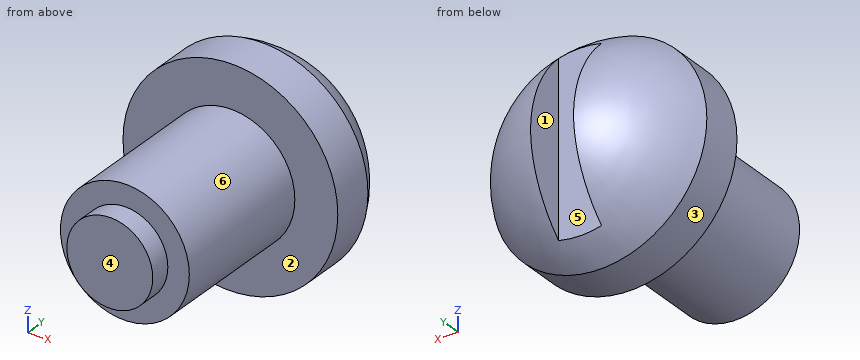
from build123d import *

# Parameters (mm, degrees)
SKETCH2_W               = 2
SKETCH2_H               = 4
CUT_EXTRUDE1_DEPTH      = 6.0000001
CUT_EXTRUDE1_DEPTH_BACK = 6.0000001


with BuildPart() as part:
    # Sketch1 → Revolve1 (revolve)
    with BuildSketch(Plane.XY):
        with BuildLine():
            Line((0, 0), (2, 0))
            Line((2, 0), (2, 1))
            Line((2, 1), (3, 1))
            Line((3, 1), (3, 8))
            Line((3, 8), (5, 8))
            Line((5, 8), (5, 10))
            ThreePointArc((5, 10), (2.938358294, 12.309260763), (0, 13.283479594))
            Line((0, 13.283479594), (0, 0))
        make_face()
    revolve(axis=Axis((0, 13.283479594, 0), (0, -1, 0)))

    # Sketch2 → Cut-Extrude1 (cut, two sides)
    with BuildSketch(Plane.XY) as cut_extrude1_sk:
        with Locations((0, 13.283479594)):
            Rectangle(SKETCH2_W, SKETCH2_H)
    extrude(amount=CUT_EXTRUDE1_DEPTH, mode=Mode.SUBTRACT)
    extrude(cut_extrude1_sk.sketch, amount=-CUT_EXTRUDE1_DEPTH_BACK, mode=Mode.SUBTRACT)


solid = part.part
Design review of the part built by this model. Coordinates are the model's own, in mm. Face numbers are marked on the shaded views. A direction names the side the tool comes from. Round coordinates to 2 decimals unless told otherwise and drop trailing zeros. Order: outer loops, then holes, each group sorted by start corner. A loop starts at its lowest first (then second) coordinate and runs counter-clockwise, first axis right, second up.
1) For L1, parallel to Y at x = 0.25, z = -4; L2, parallel to Z at x = -3, y = 9.25, list the stretches that pass through material, from the lowest coordinate up.
The answers:
L1: y = 8 to 11.28
L2: z = -4 to 4
2) Clearance check with flat-ended pins moving along their axes: pin 1 Ø4 at (x, z) = (3, 1.5) entering from +Y; pin 2 Ø5 at (y, z) = (7, 1.5) entering from +X; pin 3 Ø4 at (y, z) = (4, 1) entering from +X; pin 4 Ø4 at (x, z) = (-2.5, 4) entering from +Y. State where each tip first meets the part, or that it passes through.
The answers:
pin 1: stops at y = 13.05
pin 2: stops at x = 5
pin 3: stops at x = 3
pin 4: stops at y = 12.45
3) Draft analysis for pull direction X (two halves, no side actions). For the marked faces 4, 5 and 6, state which applies: released by +X, released by -X, zero draft, split by the parting line, or undercut.
The answers:
face 4: zero draft
face 5: undercut
face 6: split by the parting line
4) Consider section A-A (y = 6.75). State the section outline as (x, z) points, plus the area to 3 significant figures.
The answers:
outline: circle Ø6 at (0, 0)
area: 28.3 mm2
5) Machinability: for the marked faces 1, 2 and 3, which of the approach directions +Z, -Z, +X, -X, +Y, -Y give a long, thin tool a straight path to every point of the face, cutting with its end or side? Answer none if there is none.
The answers:
face 1: +Z, -Z, +Y
face 2: -Y
face 3: +Y, -Y
